```python
from build123d import *

# Parameters (mm, degrees)
F1_DEPTH     = 76.2
F2_R         = 4.7625
F3_DEPTH     = 6.35
F4_R         = 4.7625
F5_DEPTH     = 12.7
F6_R         = 3.175
F7_DEPTH     = 76.2
F8_T1_DEPTH  = 84.4391678442
F8_T3_DEPTH  = 84.0788040297
F8_T8_ANGLE  = 33.9025331494
F8_S9_R      = 4.7625
F8_T10_DEPTH = 21
F8_T14_ANGLE = 34.4766821812
F8_S15_R     = 4.7625
F8_T16_DEPTH = 21
F8_T20_ANGLE = 33.9025331494
F8_S21_R     = 4.7625
F8_T22_DEPTH = 20
F8_T26_ANGLE = 34.4766821812
F8_S27_R     = 4.7625
F8_T28_DEPTH = 20
F8_T30_ANGLE = 68.2520650555
F8_T32_ANGLE = 69.0256961544


# Not quite as in the source:
# - a fillet or chamfer that OpenCascade refuses, or shapes differently, is made with other operations: its cross-section is extruded or revolved along the edge and cut away or added


with BuildPart() as f1:
    # F0 (on Front) → F1 (new body)
    with BuildSketch(Plane.XZ):
        with BuildLine():
            Line((0, 50.8), (0, 55.5625))
            ThreePointArc((0, 55.5625), (-27.78125, 48.1185364978), (-48.1185364978, 27.78125))
            Line((-48.1185364978, 27.78125), (-43.9940905122, 25.4))
            ThreePointArc((-43.9940905122, 25.4), (-25.4, 43.9940905122), (0, 50.8))
        make_face()
    extrude(amount=F1_DEPTH)

    # F2 (on face) → F3 (join, symmetric)
    with BuildSketch(Plane.XZ.offset(76.2)):
        with Locations((-26.590625, 46.056313505)):
            Circle(F2_R)
    extrude(amount=F3_DEPTH, both=True)

    # F4 (on face) → F5 (join)
    with BuildSketch(Plane.XZ.offset(82.55)):
        with Locations((-26.590625, 46.056313505)):
            Circle(F4_R)
    extrude(amount=F5_DEPTH)

    # F6 (on face) → F7 (join)
    with BuildSketch(Plane.XZ.offset(95.25)):
        with Locations((-26.590625, 46.056313505)):
            Circle(F6_R)
    extrude(amount=F7_DEPTH)

    # F8: fillet of radius 1.6002 on 10 edges, made by hand

    # F8_s2 → F8_t1 (cut)
    with BuildSketch(Plane.XZ.offset(-4.1195839221)):
        with BuildLine():
            ThreePointArc((-46.7121706404, 26.9692842937), (-47.4637166662, 27.9639017102), (-47.2735488472, 29.1959412529))
            ThreePointArc((-47.2735488472, 29.1959412529), (-47.7012874507, 28.4917283049), (-48.1185364978, 27.78125))
            Line((-48.1185364978, 27.78125), (-46.7121706404, 26.9692842937))
        make_face()
        with BuildLine():
            ThreePointArc((-1.6476523888, 55.5380648552), (-0.4855909368, 55.0867352461), (0, 53.9385685873))
            Line((0, 53.9385685873), (0, 55.5625))
            ThreePointArc((0, 55.5625), (-0.8239167844, 55.5563908779), (-1.6476523888, 55.5380648552))
        make_face()
    extrude(amount=F8_T1_DEPTH, mode=Mode.SUBTRACT)

    # F8_s4 → F8_t3 (cut)
    with BuildSketch(Plane.XZ.offset(-3.9394020148)):
        with BuildLine():
            ThreePointArc((-45.3587394005, 26.187880403), (-44.1681291542, 26.0218753898), (-43.197905381, 26.7316473622))
            ThreePointArc((-43.197905381, 26.7316473622), (-43.6010820753, 26.0688634556), (-43.9940905122, 25.4))
            Line((-43.9940905122, 25.4), (-45.3587394005, 26.187880403))
        make_face()
        with BuildLine():
            ThreePointArc((-1.5513330102, 50.7763071313), (-0.4515405646, 51.2616595801), (0, 52.3757608059))
            Line((0, 52.3757608059), (0, 50.8))
            ThreePointArc((0, 50.8), (-0.7757569627, 50.7940764375), (-1.5513330102, 50.7763071313))
        make_face()
    extrude(amount=F8_T3_DEPTH, mode=Mode.SUBTRACT)


with BuildPart() as f8_tool6:
    # F8_s7 → F8_t8 (revolve)
    with BuildSketch(Plane(origin=(0, 0, 0), x_dir=(0, 1, 0), z_dir=(0.8640737071, 0, 0.5033653034))):
        with BuildLine():
            ThreePointArc((-74.5998, 55.5625), (-75.7313122713, 55.0938122713), (-76.2, 53.9623))
            Line((-76.2, 53.9623), (-76.2, 55.5625))
            Line((-76.2, 55.5625), (-74.5998, 55.5625))
        make_face()
    revolve(axis=Axis((0, -76.2, 0), (0, -1, 0)), revolution_arc=F8_T8_ANGLE)

    # F8_s9 → F8_t10 (cut, symmetric)
    with BuildSketch(Plane.XZ.offset(75.4)):
        with Locations((-26.590625, 46.056313505)):
            Circle(F8_S9_R)
    extrude(amount=F8_T10_DEPTH, both=True, mode=Mode.SUBTRACT)


with BuildPart() as f1_1:
    add(f1.part)

    # F8_t5: cut F8_tool6
    add(f8_tool6.part, mode=Mode.SUBTRACT)


with BuildPart() as f8_tool12:
    # F8_s13 → F8_t14 (revolve)
    with BuildSketch(Plane(origin=(0, 0, 0), x_dir=(0, 1, 0), z_dir=(-0.4303190954, 0, -0.9026768393))):
        with BuildLine():
            ThreePointArc((-74.5998, -50.8), (-75.7313122713, -51.2686877287), (-76.2, -52.4002))
            Line((-76.2, -52.4002), (-76.2, -50.8))
            Line((-76.2, -50.8), (-74.5998, -50.8))
        make_face()
    revolve(axis=Axis((0, -76.2, 0), (0, 1, 0)), revolution_arc=F8_T14_ANGLE)

    # F8_s15 → F8_t16 (cut, symmetric)
    with BuildSketch(Plane.XZ.offset(74.8)):
        with Locations((-26.590625, 46.056313505)):
            Circle(F8_S15_R)
    extrude(amount=F8_T16_DEPTH, both=True, mode=Mode.SUBTRACT)


with BuildPart() as f1_2:
    add(f1_1.part)

    # F8_t11: cut F8_tool12
    add(f8_tool12.part, mode=Mode.SUBTRACT)


with BuildPart() as f8_tool18:
    # F8_s19 → F8_t20 (revolve)
    with BuildSketch(Plane(origin=(0, 0, 0), x_dir=(0, 1, 0), z_dir=(0.9974089506, 0, -0.071940151))):
        with BuildLine():
            ThreePointArc((-74.5998, 55.5625), (-75.7313122713, 55.0938122713), (-76.2, 53.9623))
            Line((-76.2, 53.9623), (-76.2, 55.5625))
            Line((-76.2, 55.5625), (-74.5998, 55.5625))
        make_face()
    revolve(axis=Axis((0, -76.2, 0), (0, -1, 0)), revolution_arc=F8_T20_ANGLE)

    # F8_s21 → F8_t22 (cut, symmetric)
    with BuildSketch(Plane.XZ.offset(75.4)):
        with Locations((-26.590625, 46.056313505)):
            Circle(F8_S21_R)
    extrude(amount=F8_T22_DEPTH, both=True, mode=Mode.SUBTRACT)


with BuildPart() as f1_3:
    add(f1_2.part)

    # F8_t17: cut F8_tool18
    add(f8_tool18.part, mode=Mode.SUBTRACT)


with BuildPart() as f8_tool24:
    # F8_s25 → F8_t26 (revolve)
    with BuildSketch(Plane(origin=(0, 0, 0), x_dir=(0, 1, 0), z_dir=(-0.8663350804, 0, -0.4994632404))):
        with BuildLine():
            ThreePointArc((-74.5998, -50.8), (-75.7313122713, -51.2686877287), (-76.2, -52.4002))
            Line((-76.2, -52.4002), (-76.2, -50.8))
            Line((-76.2, -50.8), (-74.5998, -50.8))
        make_face()
    revolve(axis=Axis((0, -76.2, 0), (0, 1, 0)), revolution_arc=F8_T26_ANGLE)

    # F8_s27 → F8_t28 (cut, symmetric)
    with BuildSketch(Plane.XZ.offset(74.8)):
        with Locations((-26.590625, 46.056313505)):
            Circle(F8_S27_R)
    extrude(amount=F8_T28_DEPTH, both=True, mode=Mode.SUBTRACT)


with BuildPart() as f1_4:
    add(f1_3.part)

    # F8_t23: cut F8_tool24
    add(f8_tool24.part, mode=Mode.SUBTRACT)

    # F8_s29 → F8_t30 (revolve, cut)
    with BuildSketch(Plane(origin=(0, 0, 0), x_dir=(0, 1, 0), z_dir=(0.9974081949, 0, -0.0719506275))):
        with BuildLine():
            ThreePointArc((-1.6002, 55.5625), (-0.4686877287, 55.0938122713), (0, 53.9623))
            Line((0, 53.9623), (0, 55.5625))
            Line((0, 55.5625), (-1.6002, 55.5625))
        make_face()
    revolve(axis=Axis((0, 0, 0), (0, -1, 0)), revolution_arc=F8_T30_ANGLE, mode=Mode.SUBTRACT)

    # F8_s31 → F8_t32 (revolve, cut)
    with BuildSketch(Plane(origin=(0, 0, 0), x_dir=(0, 1, 0), z_dir=(-0.4303086891, 0, -0.9026818))):
        with BuildLine():
            ThreePointArc((-1.6002, -50.8), (-0.4686877287, -51.2686877287), (0, -52.4002))
            Line((0, -52.4002), (0, -50.8))
            Line((0, -50.8), (-1.6002, -50.8))
        make_face()
    revolve(axis=Axis((0, 0, 0), (0, 1, 0)), revolution_arc=F8_T32_ANGLE, mode=Mode.SUBTRACT)


solid = f1_4.part
```
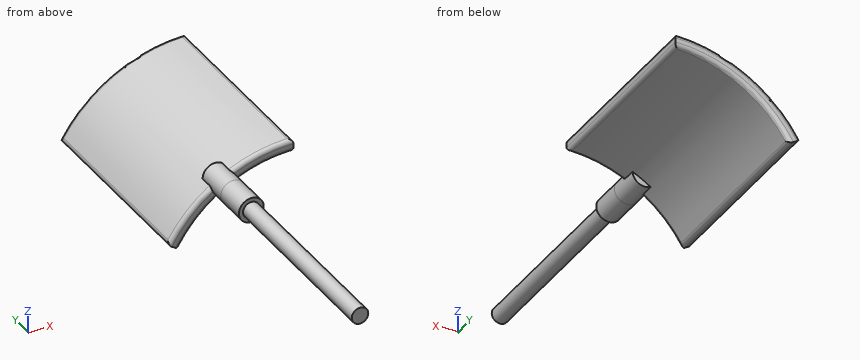
For this review, take the finished solid that the model builds, in its own axes (mm). Round coordinates to 2 decimals unless told otherwise and drop trailing zeros. Loops run counter-clockwise (first coordinate to the right, second up) from the corner with the lowest first, then second, coordinate; pieces in that order, holes last.
(1) We need section A-A (y = -72). Give the boundary of the cut face in (x, z) (1 decimal), plus the area to 3 significant figures.
Returned:
outline: (-47.3, 29.2) arc R1.6 ccw to (-46.7, 27) - (-45.4, 26.2) arc R1.6 ccw to (-43.2, 26.7) arc R50.8 cw to (-28.8, 41.8) arc R4.8 ccw to (-21.8, 45.9) arc R50.8 cw to (-1.6, 50.8) arc R1.6 ccw to (0, 52.4) - (0, 53.9) arc R1.6 ccw to (-1.6, 55.5) arc R55.6 ccw to (-24.1, 50.1) arc R4.8 ccw to (-31.3, 45.9) arc R55.6 ccw to start
area: 291 mm2
(2) Clearance check with flat-ended pins moving along their axes: P1, Ø3, axis at x = -8, z = 51, coming from the -Y side; P2, Ø3, axis at y = -74.5, z = 32, coming from the +X side; P3, Ø5.5, axis at x = -27, z = 49, coming from the +Y side; P4, Ø1.4, axis at x = -26, z = 42.5, coming from the +Y side. State where each tip first meets the part, or that it passes through.
Returned:
P1: stops at y = -76.2
P2: stops at x = -38.19
P3: stops at y = 0
P4: stops at y = -69.85
(3) We need section C-C (y = -99). Give the boundary of the cut face in (x, z) (3 decimals).
Returned:
outline: circle Ø6.35 at (-26.591, 46.056)
(4) Wall thickness on line 1 along Y through (x, z) = (-21, 49); line 2 along Z through (x, y) = (-27, -162); line 3 along X through (y, z) = (-22.5, 38.25): over which ranges is each line inside the solid? List them lowest first.
Returned:
line 1: y = -76.2 to 0
line 2: z = 42.91 to 49.2
line 3: x = -40.3 to -33.43
(5) We need section B-B (y = -48). Give the boundary of the cut face in (x, z) (1 decimal).
Returned:
outline: (-47.3, 29.2) arc R1.6 ccw to (-46.7, 27) - (-45.4, 26.2) arc R1.6 ccw to (-43.2, 26.7) arc R50.8 cw to (-1.6, 50.8) arc R1.6 ccw to (0, 52.4) - (0, 53.9) arc R1.6 ccw to (-1.6, 55.5) arc R55.6 ccw to start
